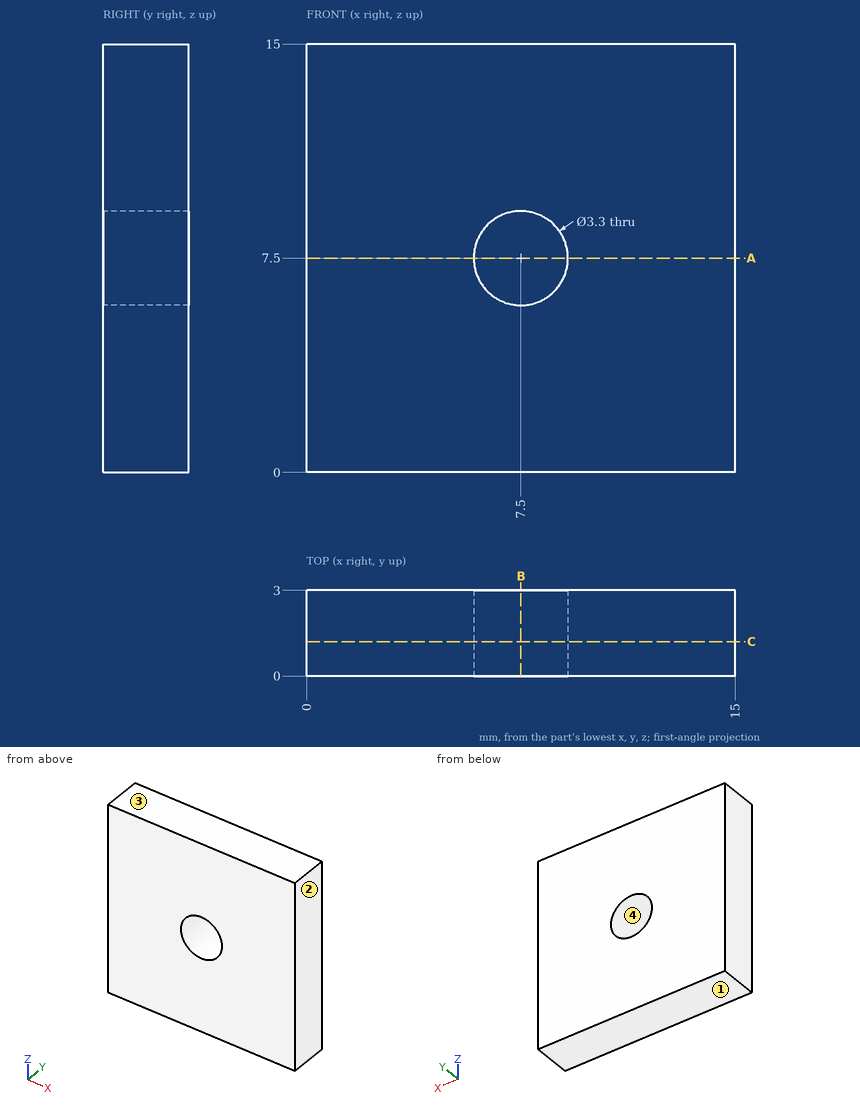
Design review of the part shown in the three views and the two pictorial views. Dimensions are in mm from the part's minimum x, y and z. Round coordinates to 2 decimals unless told otherwise and drop trailing zeros. Order: outer loops, then holes, each group sorted by start corner. A loop starts at its lowest first (then second) coordinate and runs counter-clockwise, first axis right, second up. Notation, with made-up numbers: M 66,48.25 L 98,48.25 A26 ccw 98,73.25 Z; hole C 71.25,78 d8. An arc over 180 degrees is marked long. Put each result on its own line as item: value.
Q1. Consider section C-C (y = 1.2). State the section outline as (x, z) points.
Reported:
outline: M 0,0 L 15,0 L 15,15 L 0,15 Z; hole C 7.5,7.5 d3.3
Q2. Draft analysis for pull direction Z (two halves, no side actions). For the marked faces 1, 2, 3 and 4, state which applies: released by +Z, released by -Z, zero draft, split by the parting line, or undercut.
Reported:
face 1: released by -Z
face 2: zero draft
face 3: released by +Z
face 4: undercut
Q3. Consider section A-A (z = 7.5). State the section outline as (x, y) points, and give its area (3 significant figures).
Reported:
outline: M 0,0 L 5.85,0 L 5.85,3 L 0,3 Z; M 9.15,0 L 15,0 L 15,3 L 9.15,3 Z
area: 35.1 mm²
Q4. Consider section B-B (x = 7.5). State the section outline as (y, z) points, and give its area (3 significant figures).
Reported:
outline: M 0,0 L 3,0 L 3,5.85 L 0,5.85 Z; M 0,9.15 L 3,9.15 L 3,15 L 0,15 Z
area: 35.1 mm²
Q5. To check wall thickness, follow line 1 (Z direction, x = 7.5, y = 0.8); line 2 (X direction, y = 2.8, z = 7.25); line 3 (X direction, y = 1.25, z = 6.25). State the ranges of each line that lie inside material, in increasing order.
Reported:
line 1: 0 to 5.85, 9.15 to 15
line 2: 0 to 5.87, 9.13 to 15
line 3: 0 to 6.42, 8.58 to 15
